Model file for the job. Use its own axes, mm. A direction names the side the tool comes from. Round coordinates to 2 decimals unless told otherwise and drop trailing zeros. Loops run counter-clockwise (first coordinate to the right, second up) from the corner with the lowest first, then second, coordinate; pieces in that order, holes last. Notation, with made-up numbers: (71, 40) -> (104, 40) arc R9 cw to (104, 52) -> close; hole circle Ø1 at (58, 73.5). An arc over 180 degrees is marked (long way). Use a Markdown table: item, result.
from build123d import *
from build123d.topology import SkipClean

# Parameters (mm, degrees)
REVOLVE1_ANGLE                  = 20
CIRPATTERN1_COUNT               = 2
CIRPATTERN1_ANGLE               = 7
CIRPATTERN1_THE_OTHER_WAY_COUNT = 2
CIRPATTERN1_THE_OTHER_WAY_ANGLE = 7


with BuildPart() as part:
    # Sketch2 → Revolve1 (revolve, symmetric)
    with BuildSketch(Plane(origin=(0, 0, 0), x_dir=(0, 0, -1), z_dir=(1, 0, 0))) as revolve1_sk:
        Polygon((0, 30), (2, 30), (2, 27.3), (37, 27.3), (37, 30), (4.7, 30), (4.7, 32.7), (0, 32.7), align=None)
    revolve(axis=Axis((0, 0, 0), (0, 0, -1)), revolution_arc=REVOLVE1_ANGLE / 2)
    revolve(revolve1_sk.sketch, axis=Axis((0, 0, 0), (0, 0, 1)), revolution_arc=REVOLVE1_ANGLE / 2)

    # Sketch3 → Revolve2 (revolve)
    with SkipClean():  # the faces are left unmerged after this step: merging them gives an invalid solid
        with BuildSketch(Plane(origin=(0, 0, -35.4), x_dir=(-1, 0, 0), z_dir=(0, 0, -1))):
            with BuildLine():
                Line((-1.499531177, 29.9625), (1.499531177, 29.9625))
                ThreePointArc((1.499531177, 29.9625), (0, 31.5), (-1.499531177, 29.9625))
            make_face()
        revolve2 = revolve(axis=Axis((1.499531177, 29.9625, -35.4), (-1, 0, 0)))
    add(part.part.scale(1), mode=Mode.REPLACE)  # the faces are merged on a copy

    # CirPattern1: Revolve2 ×2 about axis
    with SkipClean():  # the faces are left unmerged after this step: merging them gives an invalid solid
        cirpattern1_axis = Axis((0, 0, 0), (0, 0, -1))
        for i in range(1, CIRPATTERN1_COUNT):
            add(revolve2.rotate(cirpattern1_axis, i * CIRPATTERN1_ANGLE / (CIRPATTERN1_COUNT - 1)))
    add(part.part.scale(1), mode=Mode.REPLACE)  # the faces are merged on a copy

    # CirPattern1 the other way: Revolve2 ×2 about axis
    with SkipClean():  # the faces are left unmerged after this step: merging them gives an invalid solid
        cirpattern1_the_other_way_axis = Axis((0, 0, 0), (0, 0, 1))
        for i in range(1, CIRPATTERN1_THE_OTHER_WAY_COUNT):
            add(revolve2.rotate(cirpattern1_the_other_way_axis, i * CIRPATTERN1_THE_OTHER_WAY_ANGLE / (CIRPATTERN1_THE_OTHER_WAY_COUNT - 1)))
    add(part.part.scale(1), mode=Mode.REPLACE)  # the faces are merged on a copy

    # Mirror2: part across plane


with BuildPart() as part_1:
    add(part.part)
    add(part.part.mirror(Plane.XY))


solid = part_1.part
Q1. Drill centre lines: L1, parallel to Z at x = 3.75, y = 29.85; L2, parallel to Z at x = 4.25, y = 29.5; L3, parallel to X at y = 29.5, z = -21.5. Where is each one in solid material? Low to high. Write a range as from..to.
Results list:
| item | result |
|---|---|
| L1 | z = -36.93..-33.87, -4.7..4.7, 33.87..36.93 |
| L2 | z = -37..-2, 2..37 |
| L3 | x = -5.2..5.2 |
Q2. Band-saw the part on A-A, the plane y = 28.7. Give the cut face in (x, z).
Results list:
| item | result |
|---|---|
| outline | (-5.06, -37) -> (5.06, -37) -> (5.06, -2) -> (-5.06, -2) -> close; (-5.06, 2) -> (5.06, 2) -> (5.06, 37) -> (-5.06, 37) -> close |
Q3. Pull direction Z, two halves, no side cores. Call faces 4 (the face through (0, 28, 37)), 5 (the face through (0, 28, -37)), 6 (the face through (-5.32, 30.17, -0.52)), 7 (the face through (0, 28, 2)): released by +Z, released by -Z, zero draft, split by the parting line, or undercut.
Results list:
| item | result |
|---|---|
| face 4 | released by +Z |
| face 5 | released by -Z |
| face 6 | zero draft |
| face 7 | undercut |
Q4. Tool access for faces 1 (the face through (5.32, 30.17, -0.52)), 2 (the face through (0, 30, -17)), 3 (the face through (0, 30, 0)): list every direction of +Z, -Z, +X, -X, +Y, -Y with a clear straight run to the whole face (end or side of a thin tool).
Results list:
| item | result |
|---|---|
| face 1 | +Z, -Z, +X, -Y |
| face 2 | +Y |
| face 3 | -Y |
Q5. Flat gauge pins, fed straight in: pin 1 (5 mm diameter, centred on x = -1, z = 2, fed in from +Y); pin 2 (2.5 mm diameter, centred on x = -1.5, y = 31.5, fed in from -Z); pin 3 (4 mm diameter, centred on x = 2.5, z = 8, fed in from +Y); pin 4 (2 mm diameter, centred on y = 28.5, z = -27.5, fed in from +X). Where does each tip first touch, or does it go through?
Results list:
| item | result |
|---|---|
| pin 1 | stops at y = 32.7 |
| pin 2 | stops at z = -36.64 |
| pin 3 | stops at y = 30 |
| pin 4 | stops at x = 5.2 |
Q6. Band-saw the part on B-B, the plane z = -11.5. Give the cut face in (x, y).
Results list:
| item | result |
|---|---|
| outline | (-5.21, 29.54) -> (-4.74, 26.89) arc R27.3 cw to (4.74, 26.89) -> (5.21, 29.54) arc R30 ccw to start |
